from build123d import *

# Parameters (mm, degrees)
BOSS_EXTRUDE1_DEPTH      = 5
CUT_EXTRUDE1_DEPTH       = 10.560857702
SKETCH3_W                = 0.9
SKETCH3_H                = 0.9
CUT_EXTRUDE2_DEPTH       = 10.195860993
BOSS_EXTRUDE2_DEPTH      = 1.06
BOSS_EXTRUDE2_DEPTH_BACK = 8.94
CUT_EXTRUDE3_DEPTH       = 5.399847063
BOSS_EXTRUDE3_DEPTH      = 0.1
BOSS_EXTRUDE3_DEPTH_BACK = 2
SKETCH6_W                = 10
SKETCH6_H                = 4
SKETCH7_W                = 7
SKETCH7_H                = 2
CUT_EXTRUDE4_DEPTH       = 2
CUT_EXTRUDE4_DRAFT       = -15
CUT_EXTRUDE5_REACH       = 11.635
SKETCH9_W                = 1.06
SKETCH9_H                = 1.75
BOSS_EXTRUDE4_DEPTH      = 0.9
BOSS_EXTRUDE5_DEPTH      = 0.25
BOSS_EXTRUDE6_START      = -10.25
BOSS_EXTRUDE6_DEPTH      = 0.25


with BuildPart() as part:
    # Sketch1 → Boss-Extrude1 (new, symmetric)
    with BuildSketch(Plane(origin=(0, 0, 0), x_dir=(0, 0, -1), z_dir=(1, 0, 0))):
        Polygon((4, 7.1), (1.092777193, 7.1), (1.092777193, 6.499060719), (0, 6.499060719), (0, 0), (1.004213348, 0), (1.730924726, 0.499707627), (3.45, 0.499707627), (3.45, 5.89955469), (4, 5.89955469), align=None)
    extrude(amount=BOSS_EXTRUDE1_DEPTH, both=True)

    # Sketch2 → Cut-Extrude1 (cut, through all)
    with BuildSketch(Plane(origin=(0, 7.1, 0), x_dir=(1, 0, 0), z_dir=(0, 1, 0))):
        Polygon((-6, 4), (-4.54, 4), (-4.54, 2.85), (-3.94, 2.85), (-3.94, 2.15), (-5, 2.15), (-5, 1.75), (-3.94, 1.75), (-3.94, 0), (-6, 0), align=None)
        Polygon((6, 0), (6, 4), (4.54, 4), (4.54, 2.85), (3.94, 2.85), (3.94, 2.15), (5, 2.15), (5, 1.75), (3.94, 1.75), (3.94, 0), align=None)
    extrude(amount=-CUT_EXTRUDE1_DEPTH, mode=Mode.SUBTRACT)

    # Sketch3 → Cut-Extrude2 (cut, through all)
    with BuildSketch(Plane.XZ.offset(-0.499707627)):
        with Locations((0, -2.35)):
            Rectangle(SKETCH3_W, SKETCH3_H)
        with Locations((2.5, -2.35)):
            Rectangle(SKETCH3_W, SKETCH3_H)
        with Locations((-2.5, -2.35)):
            Rectangle(SKETCH3_W, SKETCH3_H)
    extrude(amount=-CUT_EXTRUDE2_DEPTH, mode=Mode.SUBTRACT)

    # Sketch4 → Boss-Extrude2 (add, two sides: drawn at the far end of the back side and taken through both)
    with BuildSketch(Plane(origin=(3.94, 0, 0), x_dir=(0, 0, -1), z_dir=(1, 0, 0)).offset(-BOSS_EXTRUDE2_DEPTH_BACK)):
        Polygon((1.75, 0.499707627), (1.730924726, 0.499707627), (1.4, 2.899707627), (1.75, 3.099707627), align=None)
    extrude(amount=BOSS_EXTRUDE2_DEPTH + BOSS_EXTRUDE2_DEPTH_BACK)

    # Sketch5 → Cut-Extrude3 (cut)
    with BuildSketch(Plane.XZ.offset(-0.499707627)):
        Polygon((-1.55, -3.45), (-1.25, -3.15), (-0.95, -3.45), align=None)
        Polygon((0.95, -3.45), (1.55, -3.45), (1.25, -3.15), align=None)
    extrude(amount=-CUT_EXTRUDE3_DEPTH, mode=Mode.SUBTRACT)

    # Sketch6 → Boss-Extrude3 (add, two sides: drawn at the far end of the back side and taken through both)
    with BuildSketch(Plane(origin=(0, 7.1, 0), x_dir=(1, 0, 0), z_dir=(0, 1, 0)).offset(-BOSS_EXTRUDE3_DEPTH_BACK)):
        with Locations((0, 2)):
            Rectangle(SKETCH6_W, SKETCH6_H)
    extrude(amount=BOSS_EXTRUDE3_DEPTH + BOSS_EXTRUDE3_DEPTH_BACK)


with BuildPart() as cut_extrude4_tool:
    # Sketch7 → Cut-Extrude4 (with draft: the straight prism first)
    with BuildSketch(Plane(origin=(0, 7.2, 0), x_dir=(1, 0, 0), z_dir=(0, 1, 0))):
        with Locations((0, 2.35)):
            Rectangle(SKETCH7_W, SKETCH7_H)
    extrude(amount=-CUT_EXTRUDE4_DEPTH)
    # Cut-Extrude4: the draft: its side faces are tilted about the plane it starts from
    cut_extrude4_sides = [cut_extrude4_tool.faces().sort_by_distance(p)[0] for p in [
        (-3.5, 6.2, -2.35),
        (0, 6.2, -1.35),
        (3.5, 6.2, -2.35),
        (0, 6.2, -3.35),
    ]]
    draft(cut_extrude4_sides, Plane(origin=(0, 7.2, 0), x_dir=(1, 0, 0), z_dir=(0, 1, 0)), CUT_EXTRUDE4_DRAFT)


with BuildPart() as part_1:
    add(part.part)

    # Cut-Extrude4: cut by cut_extrude4_tool
    add(cut_extrude4_tool.part, mode=Mode.SUBTRACT)

    # Cut-Extrude5: up to this face of the body (flat: up to its plane)
    cut_extrude5_end = Plane(part_1.part.faces().sort_by_distance((0, 6.22763459, -1.610544526))[0])
    # Sketch8 → Cut-Extrude5 (cut, up to the picked face)
    with BuildSketch(Plane.XY, mode=Mode.PRIVATE) as cut_extrude5_sk1:
        Polygon((-3.5, 7.2), (-2.964101615, 5.2), (2.964101615, 5.2), (3.5, 7.2), align=None)
    cut_extrude5_tool1 = split(extrude(cut_extrude5_sk1.sketch, amount=-CUT_EXTRUDE5_REACH, mode=Mode.PRIVATE), bisect_by=cut_extrude5_end, keep=Keep.BOTH, mode=Mode.PRIVATE)
    add(cut_extrude5_tool1.solids().sort_by(Axis((0, 6.227635, 0), (0, 0, -1)))[0], mode=Mode.SUBTRACT)

    # Sketch9 → Boss-Extrude4 (add)
    with BuildSketch(Plane.XZ.offset(-5.1)):
        with Locations((-4.47, -0.875)):
            Rectangle(SKETCH9_W, SKETCH9_H)
        with Locations((4.47, -0.875)):
            Rectangle(SKETCH9_W, SKETCH9_H)
    extrude(amount=BOSS_EXTRUDE4_DEPTH)

    # Sketch10 → Boss-Extrude5 (add)
    with BuildSketch(Plane(origin=(5, 0, 0), x_dir=(0, 0, -1), z_dir=(1, 0, 0))):
        Polygon((0, 4.2), (2.15, 4.2), (2.15, 5.1), (4, 5.1), (4, 7.2), (0, 7.2), align=None)
    extrude(amount=BOSS_EXTRUDE5_DEPTH)

    # Sketch10<2> → Boss-Extrude6 (add)
    with BuildSketch(Plane(origin=(5, 0, 0), x_dir=(0, 0, -1), z_dir=(1, 0, 0)).offset(BOSS_EXTRUDE6_START)):
        Polygon((0, 4.2), (2.15, 4.2), (2.15, 5.1), (4, 5.1), (4, 7.2), (0, 7.2), align=None)
    extrude(amount=BOSS_EXTRUDE6_DEPTH)


solid = part_1.part
CAD build for the part. Positions are in the model's coordinates, mm. A direction names the side the tool comes from. Round coordinates to 2 decimals unless told otherwise and drop trailing zeros. Write each loop counter-clockwise with the first axis right and the second up, starting at its lowest first coordinate (ties: lowest second). Pieces come first, ordered by that corner, then holes. Notation, with made-up numbers: M -29.75,-26.75 L -20.75,-26.75 A24 cw -20.75,-9.75 Z; hole C 2,-3 d8. An arc over 180 degrees is marked long. Put each result on its own line as item: value. Start each with the question number.
1) Drill centre lines: probe 1 along Z at (x, y) = (2.25, 1); probe 2 along X at (y, z) = (2.75, -1.95); probe 3 along Z at (x, y) = (4, 4.25). Where is each one in solid material? Low to high. Write a range as [from, to].
2) Saw through at D-D, the plane y = 5.5. Write the cut outline in (x, z), and give its area (3 significant figures).
3) 3-axis set-ups, long thin cutter, end or side, ignore diameter. For faces 1 (the flat face through (-5.25, 6, -2)), 2 (the flat face through (3, 3, -3.45)), 3 (the flat face through (2.5, 2.8, -2.8)), 4 (the flat face through (0.1, 0, -0.5)), 5 (the flat face through (4.5, 3.7, -1.75)): which of +Z, -Z, +X, -X, +Y, -Y reach the whole face in a straight line?
4) Saw through at A-A, the plane y = 4. Count the separate pieces of the cut face and the enclosed holes in it, and give its area (3 significant figures).
5) Saw through at B-B, the plane z = -0.45. Write the cut outline in (x, y).
6) Pull direction Y, two halves, no side cores. Call faces 6 (the flat face through (-4.5, 3.7, -1.75)), 7 (the flat face through (-4.48, 1.68, -1.57)), 8 (the flat face through (0, 3, -1.9)): pulls with the +Y half, pulls with the -Y half, needs draft (parallel to the pull), parting line crosses it, or undercut.
7) Pin check, flat tips, straight feed: pin 1 Ø1.5 at (y, z) = (1, -2) entering from +X; pin 2 Ø0.7 at (y, z) = (3.5, -3) entering from +X; pin 3 Ø1.5 at (x, z) = (1, -2) entering from -Y; pin 4 Ø1 at (x, y) = (-1.5, 5) entering from +Z. Stop position of each tip, or through.
8) Saw through at C-C, the plane x = -0.75. Write the cut outline in (y, z).
Resolved:
1. probe 1: [-3.45, -2.8], [-1.9, 0]
1. probe 2: [-5, -2.95], [-2.05, -0.45], [0.45, 2.05], [2.95, 5]
1. probe 3: [-3.45, -2.85], [-2.15, 0]
2. outline: M -5.25,-4 L 5.25,-4 L 5.25,0 L 3.04,0 L 3.04,-2.89 L -3.04,-2.89 L -3.04,0 L -5.25,0 Z
2. area: 24.4 mm²
3. face 1: +Z, -Z, -X, +Y, -Y
3. face 2: -Z, +X, -X, -Y
3. face 3: -Y
3. face 4: +Z, -Z, +X, -X, -Y
3. face 5: +Z, +X
4. separate pieces: 1
4. enclosed holes: 3
4. area: 26.1 mm²
5. outline: M -5.25,4.2 L -3.94,4.2 L -3.94,0 L 3.94,0 L 3.94,4.2 L 5.25,4.2 L 5.25,7.2 L 3.5,7.2 L 2.96,5.2 L -2.96,5.2 L -3.5,7.2 L -5.25,7.2 Z
6. face 6: undercut
6. face 7: pulls with the -Y half
6. face 8: needs draft
7. pin 1: x = 5
7. pin 2: x = 4.54
7. pin 3: y = 0.17
7. pin 4: z = 0
8. outline: M 0,-1 L 0.5,-1.73 L 0.5,-3.45 L 5.1,-3.45 L 5.1,-4 L 7.2,-4 L 7.2,-3.35 L 5.2,-2.81 L 5.2,0 L 0,0 Z
